CAD build for the part. Positions are in the model's coordinates, mm. Face numbers are marked on the shaded views. Coordinates: 2 decimals unless noted, no trailing zeros. Loops run counter-clockwise (first coordinate to the right, second up) from the corner with the lowest first, then second, coordinate; pieces in that order, holes last.
1) Pin check, flat tips, straight feed: pin 1 Ø0.7 at (x, y) = (-4, 11.5) entering from -Z; pin 2 Ø8 at (x, y) = (0, -8) entering from +Z; pin 3 Ø1.5 at (x, y) = (1, 7) entering from -Z; pin 4 Ø4.5 at (x, y) = (0, 8) entering from +Z. Stop position of each tip, or through.
2) Two-plate mould, pull along Y, no slides. Class the marked faces 1, 2, 3 and 4: +Y half, -Y half, draft (parallel to the pull), parting line (faces both ways), or undercut.
3) Wall check: line 1 along Y through (x, z) = (4, 2.6); line 2 along Y through (x, z) = (3.5, 3); line 3 along Y through (x, z) = (-4, 0.85). Give the ranges that are in metal, low to high.
4) Saw through at B-B, the plane y = 8. Write the cut outline in (x, z), and give its area (3 significant figures).
5) Saw through at C-C, the plane z = 2.65. Give the number of separate pieces and of enclosed holes in the cut face, and give its area (3 significant figures).
6) Saw through at A-A, the plane z = 4. Write the cut outline in (x, y).
Autodesk Inventor part; units mm, degrees
ref_plane "YZ Plane" through (0, 0, 0) normal (1, 0, 0) x (0, 1, 0)
ref_plane "XZ Plane" through (0, 0, 0) normal (0, 1, 0) x (-1, 0, 0)
ref_plane "XY Plane" through (0, 0, 0) normal (0, 0, 1) x (1, 0, 0)
sketch "Sketch1" plane through (0, 0, 0) normal (0, 0, 1) x (1, 0, 0)
  line L0 (-8, 16) -> (8, 16)
  line L1 (8, 16) -> (8, -16)
  line L2 (8, -16) -> (-8, -16)
  line L3 (-8, -16) -> (-8, 16)
  point P0 (0, 0)
  dimension "d0" = 16
  dimension "d1" = 32
  dimension "d2" = 8
  dimension "d3" = 16
extrude "Extrusion1" add sketch "Sketch1" along normal blind 3.2
shell "Shell1" thickness 1.5 removed faces 1 at (2.6667, 5.3333, 0)
sketch "Sketch2" plane through (0, 0, 3.2) normal (0, 0, 1) x (1, 0, 0)
  circle A0 centre (4, -12) radius 2.5
  line L0 (8, 16) -> (8, -16)
  line L1 (8, -16) -> (-8, -16)
  dimension "d7" = 5
  dimension "d10" = 4
  dimension "d11" = 4
extrude "Extrusion2" add sketch "Sketch2" along normal blind 1.6
sketch "Sketch3" plane through (6.5, -14.5, 1.7) normal (0, 0, -1) x (-1, 0, 0)
  circle A0 centre (2.5, 2.5) radius 2.5
  circle A1 centre (2.5, 2.5) radius 1.2
  point P0 (6.5, 14.5)
  dimension "d18" = 2.4
extrude "Extrusion3" cut sketch "Sketch3" against normal blind 1.6 contours A1
pattern_linear "Rectangular Pattern1" count 4 spacing 8 along (0, 1, 0) count 2 spacing 8 along (-1, 0, 0) of "Extrusion2", "Extrusion3"
sketch "Sketch4" plane through (6.5, -14.5, 1.7) normal (0, 0, -1) x (-1, 0, 0)
  circle A0 centre (2.5, 10.5) radius 1.2
  circle A1 centre (2.5, 2.5) radius 1.2
  line L0 (0, 29) -> (0, 0)
  line L1 (0, 0) -> (13, 0)
  circle A2 centre (6.5, 6.5) radius 3.15
  circle A3 centre (6.5, 6.5) radius 2.5
  point P0 (6.5, 14.5)
  dimension "d21" = 6.5
  dimension "d22" = 6.5
  dimension "d23" = 10.5
  dimension "d24" = 2.5
  dimension "d25" = 5
  dimension "d26" = 6.3
extrude "Extrusion4" add sketch "Sketch4" along normal up to surface (1.7 mm away) contours A2
pattern_linear "Rectangular Pattern2" count 3 spacing 8 along (0, 1, 0) of "Extrusion4"
equation "\"d0\" = 0.8 * WIDTH"
equation "\"d1\" = 0.8 * LENGTH"
equation "\"d4\" = HEIGHT"
equation "\"d21\" = 0.5 * d23 + 0.5 * d24"
equation "\"d22\" = d21"
equation "\"WIDTH\" = 2"
equation "\"HEIGHT\" = 3.2"
properties part number "3020" material "Steel"
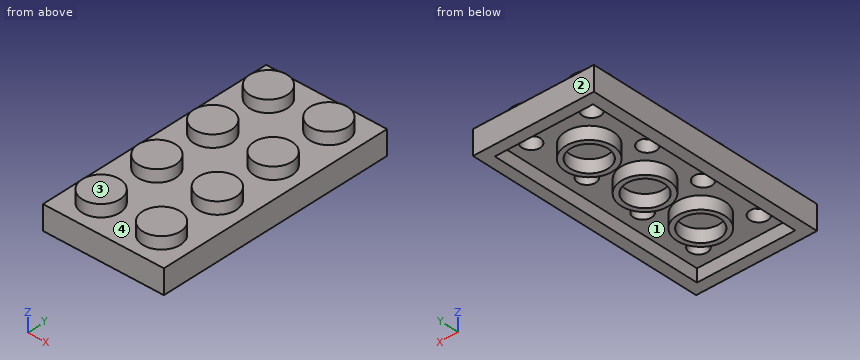
Data:
1. pin 1: stops at z = 3.3
1. pin 2: stops at z = 4.8
1. pin 3: stops at z = 1.7
1. pin 4: stops at z = 3.2
2. face 1: undercut
2. face 2: +Y half
2. face 3: draft
2. face 4: undercut
3. line 1: y = -16 to -13.2, -10.8 to -5.2, -2.8 to 2.8, 5.2 to 10.8, 13.2 to 16
3. line 2: y = -16 to -13.09, -10.91 to -5.09, -2.91 to 2.91, 5.09 to 10.91, 13.09 to 16
3. line 3: y = -16 to -14.5, 14.5 to 16
4. outline: (-8, 0) - (-6.5, 0) - (-6.5, 1.7) - (-3.15, 1.7) - (-3.15, 0) - (-2.5, 0) - (-2.5, 1.7) - (2.5, 1.7) - (2.5, 0) - (3.15, 0) - (3.15, 1.7) - (6.5, 1.7) - (6.5, 0) - (8, 0) - (8, 3.2) - (-8, 3.2) - close
4. area: 31.3 mm2
5. separate pieces: 1
5. enclosed holes: 8
5. area: 476 mm2
6. outline: circle Ø5 at (-4, -12); circle Ø5 at (-4, -4); circle Ø5 at (-4, 4); circle Ø5 at (-4, 12); circle Ø5 at (4, -12); circle Ø5 at (4, -4); circle Ø5 at (4, 4); circle Ø5 at (4, 12)
